Verification items for the finished model (mm, model axes). A direction names the side the tool comes from. Round coordinates to 2 decimals unless told otherwise and drop trailing zeros. Write each loop counter-clockwise with the first axis right and the second up, starting at its lowest first coordinate (ties: lowest second). Pieces come first, ordered by that corner, then holes. Notation, with made-up numbers: (13, 40.5) - (17, 40.5) arc R17 ccw to (17, 58.5) - close; hole circle Ø9 at (20.5, 29). An arc over 180 degrees is marked (long way). Answer as a JSON object with one key per item and string values.
```python
from build123d import *

# Parameters (mm, degrees)
SKETCH1_R         = 101.6
EXTRUDE1_DEPTH    = 12.7
SKETCH3_R         = 3.175
EXTRUDE3_DEPTH    = 145.244271983
SKETCH4_OUTSIDE_W = 262.73
SKETCH4_OUTSIDE_H = 262.73
EXTRUDE4_DEPTH    = 145.244271983


with BuildPart() as part:
    # Sketch1 → Extrude1 (new body)
    with BuildSketch(Plane.XY):
        Circle(SKETCH1_R)
    extrude(amount=EXTRUDE1_DEPTH)

    # Sketch3 → Extrude3 (cut, through all)
    with BuildSketch(Plane.XY.offset(12.7)):
        Circle(SKETCH3_R)
        with BuildLine():
            ThreePointArc((47.625, -82.48891971), (0, -95.25), (-47.625, -82.48891971))
            ThreePointArc((-47.625, -82.48891971), (-48.787130657, -78.151789053), (-44.45, -76.989658396))
            ThreePointArc((-44.45, -76.989658396), (0, -88.9), (44.45, -76.989658396))
            ThreePointArc((44.45, -76.989658396), (48.787130657, -78.151789053), (47.625, -82.48891971))
        make_face()
    extrude(amount=-EXTRUDE3_DEPTH, mode=Mode.SUBTRACT)

    # Sketch4 outside → Extrude4 (cut, through all)
    with BuildSketch(Plane.XY.offset(12.7)):
        Rectangle(SKETCH4_OUTSIDE_W, SKETCH4_OUTSIDE_H)
        with BuildLine():
            Line((-87.988181024, 50.8), (-71.490397082, 41.275))
            ThreePointArc((-71.490397082, 41.275), (-74.46179501, -35.636267817), (-12.7, -81.567226875))
            Line((-12.7, -81.567226875), (-12.7, 31.450356454))
            ThreePointArc((-12.7, 31.450356454), (0, 44.150356454), (12.7, 31.450356454))
            Line((12.7, 31.450356454), (12.7, -81.567226875))
            ThreePointArc((12.7, -81.567226875), (74.46179501, -35.636267817), (71.490397082, 41.275))
            Line((71.490397082, 41.275), (87.988181024, 50.8))
            ThreePointArc((87.988181024, 50.8), (0, -101.6), (-87.988181024, 50.8))
        make_face(mode=Mode.SUBTRACT)
    extrude(amount=-EXTRUDE4_DEPTH, mode=Mode.SUBTRACT)


solid = part.part
```
1. Mould release check, pull along X, two halves, no side actions. Record for faces 4 (the face through (73.971, -36.644, 6.439)), 5 (the face through (-2.979, -101.556, 6.261)), 6 (the face through (0, -31, 12.7)): released by +X, released by -X, zero draft, split by the parting line, or undercut.
Completed:
{"face 4": "undercut", "face 5": "split by the parting line", "face 6": "zero draft"}
2. Cross-section at A-A (y = 0). Record the boundary of the cut face in (x, z) (3 decimals).
Completed:
{"outline": "(-101.6, 0) - (-82.55, 0) - (-82.55, 12.7) - (-101.6, 12.7) - close; (-12.7, 0) - (-3.175, 0) - (-3.175, 12.7) - (-12.7, 12.7) - close; (3.175, 0) - (12.7, 0) - (12.7, 12.7) - (3.175, 12.7) - close; (82.55, 0) - (101.6, 0) - (101.6, 12.7) - (82.55, 12.7) - close"}
3. Cross-section at D-D (y = -24). Record the boundary of the cut face in (x, z).
Completed:
{"outline": "(-98.72, 0) - (-78.98, 0) - (-78.98, 12.7) - (-98.72, 12.7) - close; (-12.7, 0) - (12.7, 0) - (12.7, 12.7) - (-12.7, 12.7) - close; (78.98, 0) - (98.72, 0) - (98.72, 12.7) - (78.98, 12.7) - close"}
4. Go/stop test with flat-tipped pins: pin 1 (3 mm diameter, centred on x = -65.5, z = 2, fed in from -Y); pin 2 (1 mm diameter, centred on y = -14, z = 10.5, fed in from +X); pin 3 (4 mm diameter, centred on x = -81, z = 6, fed in from -Y). Record where each tip stops, or that it passes through.
Completed:
{"pin 1": "stops at y = -78.91", "pin 2": "stops at x = 100.7", "pin 3": "stops at y = -63.89"}
5. Access from +Z, -Z, +X, -X, +Y, -Y to the whole of each face (thin tool, end or side, straight path). Record for faces 1 (the face through (0, -31, 0)), 2 (the face through (-12.7, -26, 6)), 3 (the face through (-74.94, -34.62, 6.44)).
Completed:
{"face 1": "-Z, +X, -X, +Y, -Y", "face 2": "+Z, -Z, +Y", "face 3": "+Z, -Z"}
6. Cross-section at C-C (z = 9.5). Count the separate pieces of the cut face and the enclosed holes in it, plus the area to 3 significant figures.
Completed:
{"separate pieces": "1", "enclosed holes": "2", "area": "9,810 mm^2"}
7. Material ranges on probe 1 along Y at (x, z) = (0, 5.5) (3 decimals); probe 2 along X at (y, z) = (-57.5, 11); probe 3 along X at (y, z) = (-65, 7.75), recorded low to high. Write a range as from..to.
Completed:
{"probe 1": "y = -101.6..-95.25, -88.9..-3.175, 3.175..44.15", "probe 2": "x = -83.76..-59.23, -12.7..12.7, 59.23..83.76", "probe 3": "x = -78.09..-50.89, -12.7..12.7, 50.89..78.09"}
8. Cross-section at B-B (x = 0). Record the boundary of the cut face in (y, z) (3 decimals).
Completed:
{"outline": "(-101.6, 0) - (-95.25, 0) - (-95.25, 12.7) - (-101.6, 12.7) - close; (-88.9, 0) - (-3.175, 0) - (-3.175, 12.7) - (-88.9, 12.7) - close; (3.175, 0) - (44.15, 0) - (44.15, 12.7) - (3.175, 12.7) - close"}
